Could you check a few things on this drawing? It's one solid part, dimensions in mm from its lowest x, y, z. Round coordinates to 2 decimals unless told otherwise and drop trailing zeros. Order: outer loops, then holes, each group sorted by start corner. A loop starts at its lowest first (then second) coordinate and runs counter-clockwise, first axis right, second up. Notation, with made-up numbers: (86, 77) -> (124, 77) arc R7 cw to (124, 84) -> close; hole circle Ø2 at (86.5, -32). An arc over 180 degrees is marked (long way). Use a Markdown table: item, result. Add a question column.
(1) I want a section at A-A, the plane z = 89. Please give me the cut outline in (x, y) (3 decimals), then the cut area to 3 significant figures.
(2) I want a section at C-C, the plane x = 6.5. Please give me the cut outline in (y, z), then the cut area to 3 significant figures.
(3) I'm going to push flat-ended pins straight in: P1, Ø6, axis at x = 7.5, z = 61, coming from the +Y side; P2, Ø1.9, axis at x = 3, y = 7, coming from the -Z side; P3, Ø2, axis at x = 63, z = 77, coming from the +Y side; P4, Ø1.5, axis at x = 52, y = 6, coming from the +Z side. Where does each tip first touch, or does it pass through?
(4) I want a section at D-D, the plane x = 52. Please give me the cut outline in (y, z).
(5) I want a section at B-B, the plane y = 8.25. Please give me the cut outline in (x, z) (3 decimals), then the cut area to 3 significant figures.
(6) If I drill on probe 1 along Y at (x, z) = (54, 38); probe 2 along Y at (x, z) = (40, 39); probe 3 along Z at (x, y) = (6.5, 7.75), over which ranges is the centre line in solid material (lowest first)?
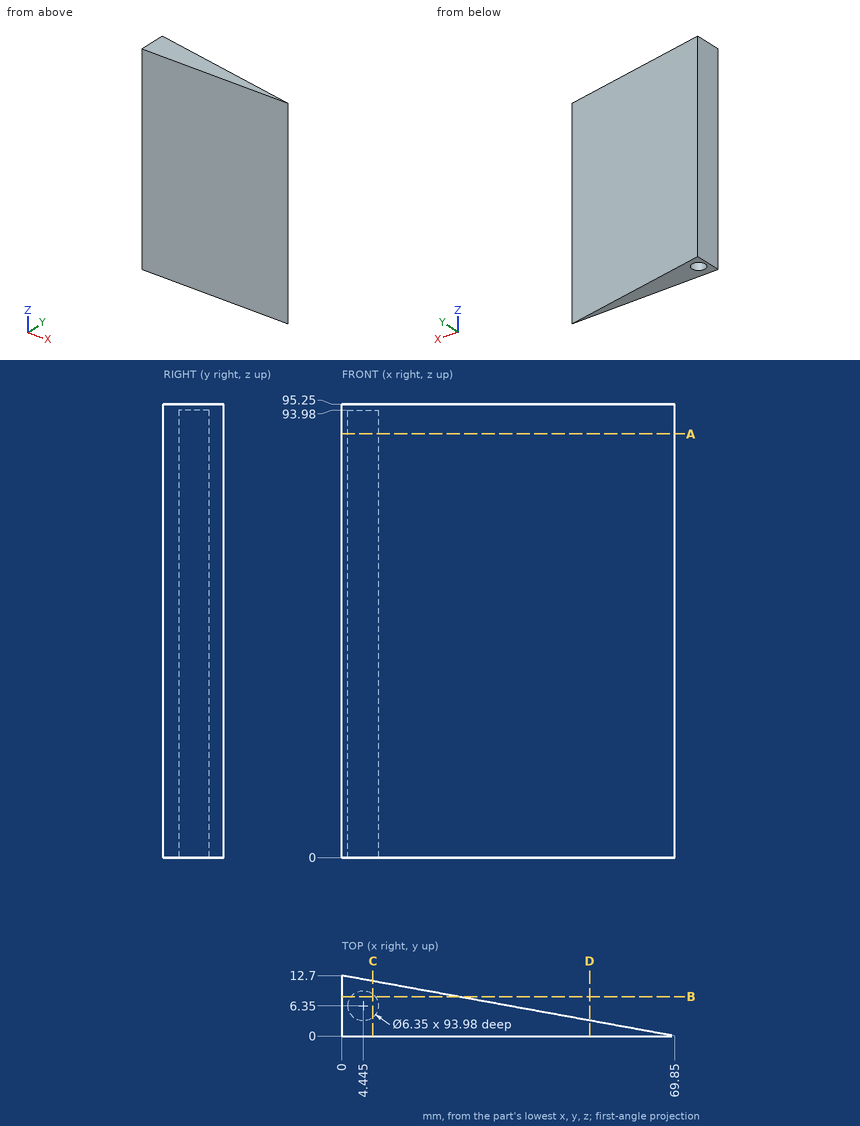
Taken from the geometry:
| question | item | result |
|---|---|---|
| 1 | outline | (0, 0) -> (69.85, 0) -> (0, 12.7) -> close; hole circle Ø6.35 at (4.445, 6.35) |
| 1 | area | 412 mm2 |
| 2 | outline | (0, 0) -> (3.93, 0) -> (3.93, 93.98) -> (8.77, 93.98) -> (8.77, 0) -> (11.52, 0) -> (11.52, 95.25) -> (0, 95.25) -> close |
| 2 | area | 642 mm2 |
| 3 | P1 | stops at y = 11.88 |
| 3 | P2 | stops at z = 93.98 |
| 3 | P3 | stops at y = 1.43 |
| 3 | P4 | passes through |
| 4 | outline | (0, 0) -> (3.25, 0) -> (3.25, 95.25) -> (0, 95.25) -> close |
| 5 | outline | (0, 0) -> (1.901, 0) -> (1.901, 93.98) -> (6.989, 93.98) -> (6.989, 0) -> (24.475, 0) -> (24.475, 95.25) -> (0, 95.25) -> close |
| 5 | area | 1,850 mm2 |
| 6 | probe 1 | y = 0 to 2.88 |
| 6 | probe 2 | y = 0 to 5.43 |
| 6 | probe 3 | z = 93.98 to 95.25 |
